from build123d import *

# Parameters (mm, degrees)
SKETCH_1_W           = 12
SKETCH_1_H           = 12
SKETCH_1_R           = 3
EXTRUDE_1_DEPTH      = 2
EXTRUDE_2_DEPTH      = 10
EXTRUDE_2_DEPTH_BACK = 2
SKETCH_2_W           = 3
SKETCH_2_H           = 12
CHAMFER_1_SIZE       = 1


with BuildPart() as part:
    # 草图1 → 凸台-拉伸1 (new body)
    with BuildSketch(Plane(origin=(0, 0, 0), x_dir=(1, 0, 0), z_dir=(0, 1, 0))):
        with Locations((6, -6)):
            Rectangle(SKETCH_1_W, SKETCH_1_H)
        with Locations(Location((6, -6, 0), (0, 0, 270))):
            Circle(SKETCH_1_R, mode=Mode.SUBTRACT)
    extrude(amount=EXTRUDE_1_DEPTH)

    # 草图2 → 凸台-拉伸2 (add, two sides: drawn at the far end of the back side and taken through both)
    with BuildSketch(Plane(origin=(0, 2, 0), x_dir=(1, 0, 0), z_dir=(0, 1, 0)).offset(-EXTRUDE_2_DEPTH_BACK)):
        with Locations((13.5, -6)):
            Rectangle(SKETCH_2_W, SKETCH_2_H)
    extrude(amount=EXTRUDE_2_DEPTH + EXTRUDE_2_DEPTH_BACK)

    # 倒角1
    chamfer_1_edges = [part.edges().sort_by_distance(p)[0] for p in [
        (6, 0, 3),
        (6, 2, 3),
        (12, 2, 6),
        (6, 2, 0),
        (12, 7, 12),
        (12, 7, 0),
        (15, 6, 0),
        (15, 0, 6),
        (15, 6, 12),
        (12, 12, 6),
        (13.5, 12, 12),
        (15, 12, 6),
        (13.5, 12, 0),
        (0, 2, 6),
        (7.5, 0, 0),
        (7.5, 0, 12),
        (0, 0, 6),
        (0, 1, 0),
        (0, 1, 12),
        (6, 2, 12),
    ]]
    chamfer(chamfer_1_edges, length=CHAMFER_1_SIZE - 0.0001)  # a hair under: the kernel refuses the full size


solid = part.part
Input: part model. Units: mm. Frame: model coordinates. A direction names the side the tool comes from. Give positions to 0.01 mm unless a question says otherwise; leave off trailing zeros. Loops run counter-clockwise (first coordinate to the right, second up) from the corner with the lowest first, then second, coordinate; pieces in that order, holes last. Notation, with made-up numbers: (19.25, 29) - (23.25, 29) arc R28 ccw to (23.25, 56) - close; hole circle Ø3 at (50, -16.5). An arc over 180 degrees is marked (long way). Use CSV: the item, a comma, the result in double quotes. Start each with the question number.
Item 1: Section D-D on x = 12.5. Return loops of the section in (y, z), then the cut area to 3 significant figures.
Item 2: Line query: line 1 (Y direction, x = 2.5, z = 9.25); line 2 (Z direction, x = 6, y = 1.05); line 3 (Z direction, x = 8, y = 1.5). Output: solid intervals per line, ascending.
Item 3: Reachability of faces 1 (the flat face through (14.5, 11.5, 6.1)), 2 (the flat face through (12.5, 6.9, 0.5)), 3 (the flat face through (12.5, 6.9, 11.5)), 4 (the flat face through (5.9, 2, 1.5)), 5 (the flat face through (14.3, 0.7, 11.4)) from +Z, -Z, +X, -X, +Y, -Y: full face, straight path, thin tool, end or side. Return the list, or none.
Item 4: Section C-C on y = 7.5. Return loops of the section in (x, z).
Item 5: Contact query for flat-ended pins moving along their axis: P1, Ø6, axis at x = 13, y = 10.5, coming from the -Z side; P2, Ø1.5, axis at x = 4, y = 3, coming from the +Z side; P3, Ø3, axis at x = 6.5, y = 2, coming from the +Z side; P4, Ø2.5, axis at y = 9, z = 3.5, coming from the -X side. Output: stop coordinate, or through.
Ans:
1,outline,"(0, 1) - (1, 0) - (2.5, 0) - (3, 0.5) - (11, 0.5) - (11.5, 1) - (11.5, 11) - (11, 11.5) - (3, 11.5) - (2.5, 12) - (1, 12) - (0, 11) - close"
1,area,"128 mm2"
2,line 1,"y = 0 to 2"
2,line 2,"z = 0.05 to 2.95, 9.05 to 11.95"
2,line 3,"z = 0.5 to 3.13, 8.87 to 11.5"
3,face 1,"+Z, -Z, +X, +Y"
3,face 2,"-Z, -X, +Y"
3,face 3,"+Z, -X, +Y"
3,face 4,"+Z, -Z, -X, +Y"
3,face 5,"+Z, +X, -Y"
4,outline,"(12, 1) - (13, 0) - (14, 0) - (15, 1) - (15, 11) - (14, 12) - (13, 12) - (12, 11) - close"
5,P1,"stops at z = 0"
5,P2,"passes through"
5,P3,"stops at z = 12"
5,P4,"stops at x = 12"
